```python
from build123d import *

# Parameters (mm, degrees)
SKETCH1_R           = 1.6
BOSS_EXTRUDE1_DEPTH = 8
CHAMFER1_SIZE       = 1


with BuildPart() as part:
    # Sketch1 → Boss-Extrude1 (new body)
    with BuildSketch(Plane.XY):
        with BuildLine():
            Line((-0.5, 3), (75.5, 3))
            ThreePointArc((75.5, 3), (77.267766953, 2.267766953), (78, 0.5))
            Line((78, 0.5), (78, -0.5))
            ThreePointArc((78, -0.5), (77.267766953, -2.267766953), (75.5, -3))
            Line((75.5, -3), (-0.5, -3))
            ThreePointArc((-0.5, -3), (-2.267766953, -2.267766953), (-3, -0.5))
            Line((-3, -0.5), (-3, 0.5))
            ThreePointArc((-3, 0.5), (-2.267766953, 2.267766953), (-0.5, 3))
        make_face()
        Circle(SKETCH1_R, mode=Mode.SUBTRACT)
        with Locations((7.5, 0)):
            Circle(SKETCH1_R, mode=Mode.SUBTRACT)
        with Locations((15, 0)):
            Circle(SKETCH1_R, mode=Mode.SUBTRACT)
        with Locations((22.5, 0)):
            Circle(SKETCH1_R, mode=Mode.SUBTRACT)
        with Locations((30, 0)):
            Circle(SKETCH1_R, mode=Mode.SUBTRACT)
        with Locations((37.5, 0)):
            Circle(SKETCH1_R, mode=Mode.SUBTRACT)
        with Locations((45, 0)):
            Circle(SKETCH1_R, mode=Mode.SUBTRACT)
        with Locations((52.5, 0)):
            Circle(SKETCH1_R, mode=Mode.SUBTRACT)
        with Locations((60, 0)):
            Circle(SKETCH1_R, mode=Mode.SUBTRACT)
        with Locations((67.5, 0)):
            Circle(SKETCH1_R, mode=Mode.SUBTRACT)
        with Locations((75, 0)):
            Circle(SKETCH1_R, mode=Mode.SUBTRACT)
    extrude(amount=BOSS_EXTRUDE1_DEPTH)

    # Chamfer1
    chamfer1_edges = [part.edges().sort_by_distance(p)[0] for p in [
        (-1.6, 0, 0),
        (-1.6, 0, 8),
        (5.9, 0, 0),
        (5.9, 0, 8),
        (13.4, 0, 0),
        (13.4, 0, 8),
        (20.9, 0, 0),
        (20.9, 0, 8),
        (28.4, 0, 0),
        (28.4, 0, 8),
        (35.9, 0, 0),
        (35.9, 0, 8),
        (43.4, 0, 0),
        (43.4, 0, 8),
        (50.9, 0, 0),
        (50.9, 0, 8),
        (58.4, 0, 0),
        (58.4, 0, 8),
        (65.9, 0, 0),
        (65.9, 0, 8),
        (73.4, 0, 0),
        (73.4, 0, 8),
    ]]
    chamfer(chamfer1_edges, length=CHAMFER1_SIZE)


solid = part.part
```
Work out the finished part from the listing and answer in its coordinate system (mm). Give positions to 0.01 mm unless a question says otherwise; leave off trailing zeros. Loops run counter-clockwise (first coordinate to the right, second up) from the corner with the lowest first, then second, coordinate; pieces in that order, holes last. Notation, with made-up numbers: (-7, -9.75) -> (40, -9.75) arc R17 cw to (40, 19.25) -> close; hole circle Ø5 at (88.5, 22). An arc over 180 degrees is marked (long way). Put each result on its own line as item: value. Start each with the question number.
Item 1: This flat-tipped pin is pushed along its axis until it touches: P1, Ø3.5, axis at x = 67.5, y = 0, coming from the -Z side. Where does it stop, or does it pass through?
Item 2: The mould has two halves that part along Y. Classify faces 1 (the face through (38, -3, 4)), 2 (the face through (5.9, 0.07, 3.96)), 3 (the face through (38.1, 2.7, 8)): released by +Y, released by -Y, zero draft, split by the parting line, or undercut.
Item 3: The part is cut by section A-A (x = 52.5). Give the vertices of the cut face in (y, z).
Item 4: The part is cut by section B-B (z = 4). State how many separate pieces and enclosed holes the cut face has, then the cut area to 3 significant figures.
Item 5: Find the intervals of material crossed by L1, parallel to Y at x = 0, z = 2.8; L2, parallel to X at y = -2.75, z = 4.75; L3, parallel to X at y = 1.7, z = 5.5, in increasing order. Write a range as [from, to].
Answers below:
1. P1: z = 0.85
2. face 1: released by -Y
2. face 2: undercut
2. face 3: zero draft
3. outline: (-3, 0) -> (-2.6, 0) -> (-1.6, 1) -> (-1.6, 7) -> (-2.6, 8) -> (-3, 8) -> close; (1.6, 1) -> (2.6, 0) -> (3, 0) -> (3, 8) -> (2.6, 8) -> (1.6, 7) -> close
4. separate pieces: 1
4. enclosed holes: 11
4. area: 392 mm2
5. L1: [-3, -1.6], [1.6, 3]
5. L2: [-1.59, 76.59]
5. L3: [-2.69, 77.69]
